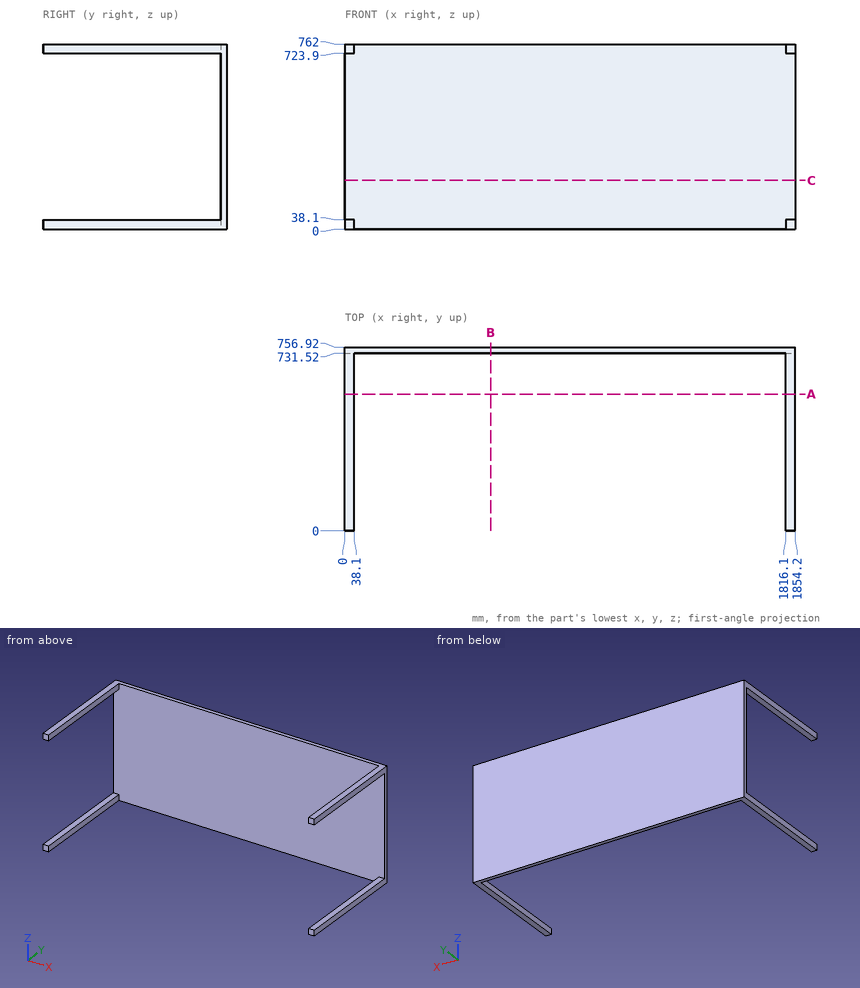
Geometry: see drawing. Coordinates: mm, zero at the bounding-box minimum. Round coordinates to 2 decimals unless told otherwise and drop trailing zeros. Order: outer loops, then holes, each group sorted by start corner. A loop starts at its lowest first (then second) coordinate and runs counter-clockwise, first axis right, second up. Notation, with made-up numbers: (33.25, 2) - (47.25, 2) arc R27 ccw to (47.25, 26) - close; hole circle Ø5 at (22, 40). An arc over 180 degrees is marked (long way). Use a Markdown table: item, result. Add a question column.
1. Section query B-B (x = 601). Return the cut outline in (y, z).
2. Line query: probe 1 along Y at (x, z) = (1102, 60). Output: solid intervals per line, ascending.
3. Section query C-C (z = 200). Return the cut outline in (x, y), then the cut area to 3 significant figures.
4. Section query A-A (y = 562.5). Return the cut outline in (x, z).
Derived:
| question | item | result |
|---|---|---|
| 1 | outline | (731.52, 0) - (756.92, 0) - (756.92, 762) - (731.52, 762) - close |
| 2 | probe 1 | 731.52 to 756.92 |
| 3 | outline | (0, 731.52) - (1854.2, 731.52) - (1854.2, 756.92) - (0, 756.92) - close |
| 3 | area | 47,100 mm2 |
| 4 | outline | (0, 0) - (38.1, 0) - (38.1, 38.1) - (0, 38.1) - close; (0, 723.9) - (38.1, 723.9) - (38.1, 762) - (0, 762) - close; (1816.1, 0) - (1854.2, 0) - (1854.2, 38.1) - (1816.1, 38.1) - close; (1816.1, 723.9) - (1854.2, 723.9) - (1854.2, 762) - (1816.1, 762) - close |
